CAD build for the part. Positions are in the model's coordinates, mm. Face numbers are marked on the shaded views. A direction names the side the tool comes from. Give positions to 0.01 mm unless a question says otherwise; leave off trailing zeros. Write each loop counter-clockwise with the first axis right and the second up, starting at its lowest first coordinate (ties: lowest second). Pieces come first, ordered by that corner, then holes. Notation, with made-up numbers: (-33.75, 38.25) - (2.25, 38.25) arc R17 ccw to (2.25, 71.25) - close; hole circle Ø1 at (70.5, -29). An arc over 180 degrees is marked (long way). Answer as a JSON object with one key per item and string values.
from build123d import *

# Parameters (mm, degrees)
SKETCH1_W                          = 16
SKETCH1_H                          = 16
SKETCH1_R                          = 3
BOSS_EXTRUDE1_DEPTH                = 6
TAP_DRILL_FOR_M2_5X0_45_TAP1_D     = 2.05
TAP_DRILL_FOR_M2_5X0_45_TAP1_DEPTH = 4.5
TAP_DRILL_FOR_M2_5X0_45_TAP1_TIP   = 0.615882135
SKETCH5_R                          = 3.1
SKETCH5_R_2                        = 1
CUT_EXTRUDE1_DEPTH                 = 19.867962264
SKETCH6_R                          = 1.5
CUT_EXTRUDE2_DEPTH                 = 6
CHAMFER1_SIZE                      = 0.5
CHAMFER2_SIZE                      = 0.25


with BuildPart() as part:
    # Sketch1 → Boss-Extrude1 (new, symmetric)
    with BuildSketch(Plane(origin=(0, 0, 0), x_dir=(1, 0, 0), z_dir=(0, 1, 0))):
        Rectangle(SKETCH1_W, SKETCH1_H)
        with Locations(Location((-4, 0, 0), (0, 0, 270))):
            Circle(SKETCH1_R, mode=Mode.SUBTRACT)
    extrude(amount=BOSS_EXTRUDE1_DEPTH, both=True)

    # Tap Drill for M2.5x0.45 Tap1
    with Locations(Plane.XY.offset(8)):
        with Locations((-6, -4)):
            Hole(TAP_DRILL_FOR_M2_5X0_45_TAP1_D / 2, depth=TAP_DRILL_FOR_M2_5X0_45_TAP1_DEPTH)
            with Locations((0, 0, -(TAP_DRILL_FOR_M2_5X0_45_TAP1_DEPTH + TAP_DRILL_FOR_M2_5X0_45_TAP1_TIP / 2))):  # 118° drill point
                Cone(0, TAP_DRILL_FOR_M2_5X0_45_TAP1_D / 2, TAP_DRILL_FOR_M2_5X0_45_TAP1_TIP, mode=Mode.SUBTRACT)

    # Sketch5 → Cut-Extrude1 (cut, through all)
    with BuildSketch(Plane.XY.offset(8)):
        with Locations((3, 1)):
            Circle(SKETCH5_R)
        with Locations((5, -4)):
            Circle(SKETCH5_R_2)
    extrude(amount=-CUT_EXTRUDE1_DEPTH, mode=Mode.SUBTRACT)

    # Sketch6 → Cut-Extrude2 (cut)
    with BuildSketch(Plane(origin=(0, 6, 0), x_dir=(1, 0, 0), z_dir=(0, 1, 0))):
        with Locations(Location((3, 0, 0), (0, 0, 270))):
            Circle(SKETCH6_R)
    extrude(amount=-CUT_EXTRUDE2_DEPTH, mode=Mode.SUBTRACT)

    # Chamfer1
    chamfer1_edges = [part.edges().sort_by_distance(p)[0] for p in [
        (8, 6, 0),
        (8, 0, 8),
        (-8, 0, 8),
        (-8, 0, -8),
        (8, 0, -8),
        (0, 6, -8),
        (-8, 6, 0),
        (0, 6, 8),
        (0, -6, 8),
        (-8, -6, 0),
        (0, -6, -8),
        (8, -6, 0),
    ]]
    chamfer(chamfer1_edges, length=CHAMFER1_SIZE)

    # Chamfer2
    chamfer2_edges = [part.edges().sort_by_distance(p)[0] for p in [
        (3, 6, -1.5),
        (-4, 6, -3),
        (-4, -6, -3),
    ]]
    chamfer(chamfer2_edges, length=CHAMFER2_SIZE)


solid = part.part
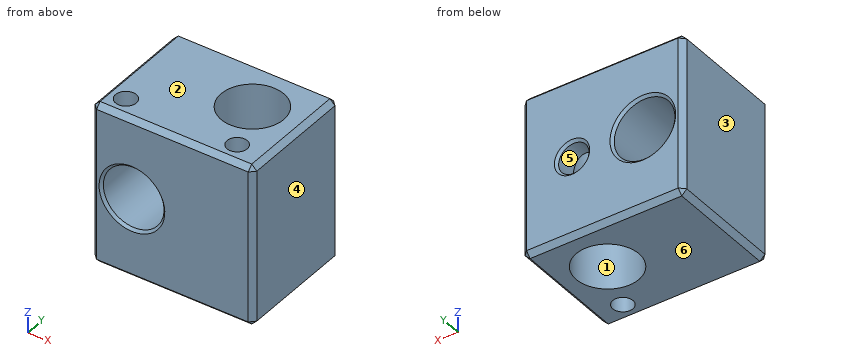
Item 1: Cut at A-A (x = 3). Give the cut face in (y, z), and give its area (3 significant figures).
Entries:
{"outline": "(-6, -7.5) - (-5.5, -8) - (-2.1, -8) - (-2.1, 8) - (-5.5, 8) - (-6, 7.5) - close; (4.1, -8) - (5.5, -8) - (6, -7.5) - (6, -1.75) - (5.75, -1.5) - (4.1, -1.5) - close; (4.1, 1.5) - (5.75, 1.5) - (6, 1.75) - (6, 7.5) - (5.5, 8) - (4.1, 8) - close", "area": "86.5 mm2"}
Item 2: Cut at C-C (y = 1). Give the cut face in (x, z), and give its area (3 significant figures).
Entries:
{"outline": "(-8, -7.5) - (-7.5, -8) - (-0.1, -8) - (-0.1, 8) - (-7.5, 8) - (-8, 7.5) - close; (6.1, -8) - (7.5, -8) - (8, -7.5) - (8, 7.5) - (7.5, 8) - (6.1, 8) - close; hole circle Ø6 at (-4, 0)", "area": "128 mm2"}
Item 3: Cut at B-B (z = 0). Give the cut face in (x, y).
Entries:
{"outline": "(-8, -5.5) - (-7.5, -6) - (-7.25, -6) - (-7, -5.75) - (-7, 5.75) - (-7.25, 6) - (-7.5, 6) - (-8, 5.5) - close; (-1, -5.75) - (-0.75, -6) - (7.5, -6) - (8, -5.5) - (8, 5.5) - (7.5, 6) - (4.75, 6) - (4.5, 5.75) - (4.5, 3.71) arc R3.1 cw (long way) to (1.5, 3.71) - (1.5, 5.75) - (1.25, 6) - (-0.75, 6) - (-1, 5.75) - close; hole circle Ø2 at (5, -4)"}
Item 4: Cut at D-D (z = 6.75). Give the cut face in (x, y) (3 decimals).
Entries:
{"outline": "(-8, -5.5) - (-7.5, -6) - (7.5, -6) - (8, -5.5) - (8, 5.5) - (7.5, 6) - (-7.5, 6) - (-8, 5.5) - close; hole circle Ø2.05 at (-6, -4); hole circle Ø6.2 at (3, 1); hole circle Ø2 at (5, -4)"}
Item 5: Flat gauge pins, fed straight in: P1, Ø2.5, axis at x = -6, y = -4, coming from the +Z side; P2, Ø3.5, axis at x = 3, y = 1, coming from the +Z side. Where does each tip first touch, or does it go through?
Entries:
{"P1": "z = 8", "P2": "through"}
Item 6: Which spindle directions (+Z, -Z, +X, -X, +Y, -Y) get a long thin tool onto all of the face, cutting with end or side? Do the marked faces 5 and 6. Say none if no direction does.
Entries:
{"face 5": "+Y", "face 6": "-Z, +X, -X, +Y, -Y"}
Item 7: Mould opens along X. For the marked faces 1, 2, 3 and 4 say: +X half, -X half, draft (parallel to the pull), parting line (faces both ways), or undercut.
Entries:
{"face 1": "undercut", "face 2": "draft", "face 3": "-X half", "face 4": "+X half"}
Item 8: Probe line 1 (X direction, y = 4.9, z = 0); line 2 (X direction, y = -3.25, z = 2.5); line 3 (Z direction, x = 3, y = 4.75). List the from-to ranges inside material, lowest first. Write a range as from..to.
Entries:
{"line 1": "-8..-7, -1..1.5, 4.5..8", "line 2": "-8..-5.66, -2.34..4.34, 5.66..8", "line 3": "-8..-1.5, 1.5..8"}
